from build123d import *

# Parameters (mm, degrees)
CROQUIS1_W              = 310.8
CROQUIS1_H              = 200.8
CROQUIS1_W_2            = 260
CROQUIS1_H_2            = 150
SALIENTE_EXTRUIR1_DEPTH = 12.7
CROQUIS2_W              = 310.8
CROQUIS2_H              = 200.8
SALIENTE_EXTRUIR2_DEPTH = 0.2


with BuildPart() as part:
    # Croquis1 → Saliente-Extruir1 (new body)
    with BuildSketch(Plane(origin=(0, 0, 0), x_dir=(1, 0, 0), z_dir=(0, 1, 0))):
        Rectangle(CROQUIS1_W, CROQUIS1_H)
        Rectangle(CROQUIS1_W_2, CROQUIS1_H_2, mode=Mode.SUBTRACT)
    extrude(amount=SALIENTE_EXTRUIR1_DEPTH)

    # Croquis2 → Saliente-Extruir2 (add)
    with BuildSketch(Plane.XZ):
        Rectangle(CROQUIS2_W, CROQUIS2_H)
    extrude(amount=SALIENTE_EXTRUIR2_DEPTH)


solid = part.part
Design review of the part built by this model. Coordinates are the model's own, in mm. A direction names the side the tool comes from. Give positions to 0.01 mm unless a question says otherwise; leave off trailing zeros. Write each loop counter-clockwise with the first axis right and the second up, starting at its lowest first coordinate (ties: lowest second). Pieces come first, ordered by that corner, then holes. Notation, with made-up numbers: M 71.5,73.5 L 107.5,73.5 A21 ccw 107.5,95.5 Z; hole C -36.75,8.5 d7. An arc over 180 degrees is marked long. Answer as a JSON object with one key per item and string values. Group by question number.
1) We need section C-C (z = 8). Give the boundary of the cut face in (x, y), and give its area (3 significant figures).
2) Clearance check with a flat-ended pin moving along its axis: pin 1 Ø6 at (x, z) = (-60.5, 16.5) entering from +Y. State where the tip first meets the part, or that it passes through.
3) We need section B-B (x = 57). Give the boundary of the cut face in (y, z), and give its area (3 significant figures).
4) We need section A-A (y = 3.5). Give the boundary of the cut face in (x, z).
5) Mouldability with a two-part tool opening along Z and no side actions: class faces 1 (the face through (-2, 6, 100.4)), 2 (the face through (-155.4, 6, -1)), 3 (the face through (-2, 6, -75)), 4 (the face through (130, 6, 1)) as released by +Z, released by -Z, zero draft, split by the parting line, or undercut.
6) Tool access review of faces 5 (the face through (-2, 6, 75)), 6 (the face through (-2, 12.7, 88)): name each direction out of +Z, -Z, +X, -X, +Y, -Y from which nothing blocks a thin tool from reaching the whole face with its end or side.
7) For line 1 along X through (y, z) = (7.5, 34.5); line 2 along Z through (x, y) = (120, 10); line 3 along Y through (x, z) = (72.5, 38.5), list the stretches that pass through material, from the lowest coordinate up.
Answer key:
{
 "1": {"outline": "M -155.4,-0.2 L 155.4,-0.2 L 155.4,12.7 L 130,12.7 L 130,0 L -130,0 L -130,12.7 L -155.4,12.7 Z", "area": "707 mm²"},
 "2": {"pin 1": "stops at y = 0"},
 "3": {"outline": "M -0.2,-100.4 L 12.7,-100.4 L 12.7,-75 L 0,-75 L 0,75 L 12.7,75 L 12.7,100.4 L -0.2,100.4 Z", "area": "685 mm²"},
 "4": {"outline": "M -155.4,-100.4 L 155.4,-100.4 L 155.4,100.4 L -155.4,100.4 Z; hole M -130,-75 L 130,-75 L 130,75 L -130,75 Z"},
 "5": {"face 1": "released by +Z", "face 2": "zero draft", "face 3": "undercut", "face 4": "undercut"},
 "6": {"face 5": "+Y", "face 6": "+Z, -Z, +X, -X, +Y"},
 "7": {"line 1": "x = -155.4 to -130, 130 to 155.4", "line 2": "z = -100.4 to -75, 75 to 100.4", "line 3": "y = -0.2 to 0"}
}
